from build123d import *

# Parameters (mm, degrees)
ESBO_O1_R                = 14
ESBO_O1_R_2              = 5
ESBO_O1_R_3              = 1.25
RESSALTO_EXTRUS_O1_DEPTH = 2.5


with BuildPart() as part:
    # Esboço1 → Ressalto-extrusão1 (new body)
    with BuildSketch(Plane.XY):
        Circle(ESBO_O1_R)
        Circle(ESBO_O1_R_2, mode=Mode.SUBTRACT)
        with Locations((0, 11)):
            Circle(ESBO_O1_R_3, mode=Mode.SUBTRACT)
        with Locations((7.778174593, 7.778174593)):
            Circle(ESBO_O1_R_3, mode=Mode.SUBTRACT)
        with Locations((11, 0)):
            Circle(ESBO_O1_R_3, mode=Mode.SUBTRACT)
        with Locations((7.778174593, -7.778174593)):
            Circle(ESBO_O1_R_3, mode=Mode.SUBTRACT)
        with Locations((0, -11)):
            Circle(ESBO_O1_R_3, mode=Mode.SUBTRACT)
        with Locations((-7.778174593, -7.778174593)):
            Circle(ESBO_O1_R_3, mode=Mode.SUBTRACT)
        with Locations((-11, 0)):
            Circle(ESBO_O1_R_3, mode=Mode.SUBTRACT)
        with Locations((-7.778174593, 7.778174593)):
            Circle(ESBO_O1_R_3, mode=Mode.SUBTRACT)
    extrude(amount=RESSALTO_EXTRUS_O1_DEPTH)


solid = part.part
Design review of the part built by this model. Coordinates are the model's own, in mm. Give positions to 0.01 mm unless a question says otherwise; leave off trailing zeros. Write each loop counter-clockwise with the first axis right and the second up, starting at its lowest first coordinate (ties: lowest second). Pieces come first, ordered by that corner, then holes. Notation, with made-up numbers: M -23.5,24.25 L 33.5,24.25 A28 ccw 33.5,58.25 Z; hole C 50,50.5 d6. An arc over 180 degrees is marked long. Answer as a JSON object with one key per item and string values. Group by question number.
1) Clearance check with flat-ended pins moving along their axes: pin 1 Ø1 at (y, z) = (8.5, 2) entering from -X; pin 2 Ø2 at (x, y) = (-7.78, -7.78) entering from +Z; pin 3 Ø2 at (x, y) = (10.5, -6.5) entering from -Z; pin 4 Ø1.5 at (x, z) = (-3.5, 1) entering from +Y. State where each tip first meets the part, or that it passes through.
2) We need section D-D (z = 1.2). Count the separate pieces of the cut face and the enclosed holes in it, and give its area (3 significant figures).
3) We need section C-C (x = -8.25). Give the boundary of the cut face in (y, z).
4) We need section A-A (x = 0). Give the boundary of the cut face in (y, z), and give its area (3 significant figures).
5) Mouldability with a two-part tool opening along Y and no side actions: class faces 1 (the face through (0, -6, 2.5)), 2 (the face through (-1.08, -4.88, 1.23)), 3 (the face through (-7.941, 9.018, 1.232)), 4 (the face through (12.932, -5.362, 1.232)) as released by +Y, released by -Y, zero draft, split by the parting line, or undercut.
6) For line 1 along X through (y, z) = (-8.5, 1.35); line 2 along Y through (x, z) = (-8.75, 1.3); line 3 along Y through (x, z) = (11.5, 2.45), list the stretches that pass through material, from the lowest coordinate up.
Answer key:
{
 "1": {"pin 1": "stops at x = -11.49", "pin 2": "passes through", "pin 3": "stops at z = 0", "pin 4": "stops at y = 13.73"},
 "2": {"separate pieces": "1", "enclosed holes": "9", "area": "498 mm²"},
 "3": {"outline": "M -11.31,0 L -8.94,0 L -8.94,2.5 L -11.31,2.5 Z; M -6.62,0 L 6.62,0 L 6.62,2.5 L -6.62,2.5 Z; M 8.94,0 L 11.31,0 L 11.31,2.5 L 8.94,2.5 Z"},
 "4": {"outline": "M -14,0 L -12.25,0 L -12.25,2.5 L -14,2.5 Z; M -9.75,0 L -5,0 L -5,2.5 L -9.75,2.5 Z; M 5,0 L 9.75,0 L 9.75,2.5 L 5,2.5 Z; M 12.25,0 L 14,0 L 14,2.5 L 12.25,2.5 Z", "area": "32.5 mm²"},
 "5": {"face 1": "zero draft", "face 2": "undercut", "face 3": "undercut", "face 4": "split by the parting line"},
 "6": {"line 1": "x = -11.12 to -8.8, -6.76 to 6.76, 8.8 to 11.12", "line 2": "y = -10.93 to -8.56, -6.99 to 6.99, 8.56 to 10.93", "line 3": "y = -7.98 to -1.15, 1.15 to 7.98"}
}
